Source: CAD feature listing. Evaluate the final solid. Frame: model axes, mm. A direction names the side the tool comes from. Give positions to 0.01 mm unless a question says otherwise; leave off trailing zeros. Write each loop counter-clockwise with the first axis right and the second up, starting at its lowest first coordinate (ties: lowest second). Pieces come first, ordered by that corner, then holes. Notation, with made-up numbers: (33.5, -14.5) -> (64.5, -14.5) arc R6 cw to (64.5, -10.5) -> close; hole circle Ø2 at (67, 28.25). An arc over 180 degrees is marked (long way). Write item = value, one per line.
from build123d import *

# Parameters (mm, degrees)
SKETCH_2_R               = 1.5
CUT_EXTRUDE_1_DEPTH      = 10
PATTERN_CIRCULAR_1_COUNT = 4
CUT_EXTRUDE_3_REACH      = 41.211
SKETCH_3_R               = 3.5
CUT_EXTRUDE_4_REACH      = 41.211
CUT_EXTRUDE_4_END_RADIUS = 1.5
SKETCH_4_W               = 31.367872694
SKETCH_4_H               = 2
CUT_EXTRUDE_START        = -24
SKETCH_5_W               = 2
SKETCH_5_H               = 28.424190946
CUT_EXTRUDE_5_DEPTH      = 24


with BuildPart() as part:
    # 草图1 → 旋转1 (revolve)
    with BuildSketch(Plane(origin=(0, 0, 0), x_dir=(0, 0, -1), z_dir=(1, 0, 0)), mode=Mode.PRIVATE) as revolve_1_sk:
        Polygon((-2.5, 6.5), (2.5, 6.5), (2.5, 9), (8.5, 9), (8.5, 0), (-26.5, 0), (-26.5, 9), (-22.5, 9), (-22.5, 12.5), (-2.5, 9.653578486), align=None)
    revolve(revolve_1_sk.sketch.rotate(Axis((0, 0, 115.12599891), (0, 0, -1)), 90), axis=Axis((0, 0, 115.12599891), (0, 0, -1)))

    # 草图2 → 切除-拉伸1 (cut)
    with BuildSketch(Plane(origin=(0, 0, 0), x_dir=(1, 0, 0), z_dir=(0, 1, 0))):
        with Locations(Location((0, 0, 0), (0, 0, 270))):
            Circle(SKETCH_2_R)
    cut_extrude_1 = extrude(amount=-CUT_EXTRUDE_1_DEPTH, mode=Mode.SUBTRACT)

    # 阵列(圆周)1: 切除-拉伸1 ×4 about axis
    pattern_circular_1_axis = Axis((0, 0, 2.5), (0, 0, 1))
    for i in range(1, PATTERN_CIRCULAR_1_COUNT):
        add(cut_extrude_1.rotate(pattern_circular_1_axis, i * 360 / PATTERN_CIRCULAR_1_COUNT), mode=Mode.SUBTRACT)

    # 草图3 → 切除-拉伸3 (cut, up to next)
    with BuildSketch(Plane(origin=(0, 0, -8.5), x_dir=(-1, 0, 0), z_dir=(0, 0, -1)), mode=Mode.PRIVATE) as cut_extrude_3_sk1:
        Circle(SKETCH_3_R)
    cut_extrude_3_tool1 = extrude(cut_extrude_3_sk1.sketch, amount=-CUT_EXTRUDE_3_REACH, mode=Mode.PRIVATE) & part.part
    add(cut_extrude_3_tool1.solids().sort_by_distance((0, 0, -8.5))[0], mode=Mode.SUBTRACT)

    # 切除-拉伸4: up to this cylinder (the profile starts outside it)
    cut_extrude_4_end = Plane(origin=(0, 0, 0), z_dir=(-1, 0, 0)) * Cylinder(CUT_EXTRUDE_4_END_RADIUS, 86.422, mode=Mode.PRIVATE)
    # 草图4 → 切除-拉伸4 (cut, up to the surface)
    with BuildSketch(Plane.XY.offset(26.5), mode=Mode.PRIVATE) as cut_extrude_4_sk1:
        Rectangle(SKETCH_4_W, SKETCH_4_H)
    cut_extrude_4_tool1 = extrude(cut_extrude_4_sk1.sketch, amount=-CUT_EXTRUDE_4_REACH, mode=Mode.PRIVATE) - cut_extrude_4_end
    add(cut_extrude_4_tool1.solids().sort_by_distance((0, 0, 26.5))[0], mode=Mode.SUBTRACT)

    # 草图5 → 切除-拉伸5 (cut)
    with BuildSketch(Plane.XY.offset(26.5).offset(CUT_EXTRUDE_START)):
        Rectangle(SKETCH_5_W, SKETCH_5_H)
    extrude(amount=CUT_EXTRUDE_5_DEPTH, mode=Mode.SUBTRACT)


solid = part.part
(1) Section query A-A (x = 0). Return loops of the section in (y, z).
Values follow:
outline = (-9, -8.5) -> (-3.5, -8.5) -> (-3.5, -1.5) -> (-6.5, -1.5) -> (-6.5, -2.5) -> (-9, -2.5) -> close; (-6.5, 1.5) -> (-3.5, 1.5) -> (-3.5, 2.5) -> (-6.5, 2.5) -> close; (3.5, -8.5) -> (9, -8.5) -> (9, -2.5) -> (6.5, -2.5) -> (6.5, -1.5) -> (3.5, -1.5) -> close; (3.5, 1.5) -> (6.5, 1.5) -> (6.5, 2.5) -> (3.5, 2.5) -> close
(2) First-contact query: pin 1 (4 mm diameter, centred on x = 0, z = 0, fed in from +Y); pin 2 (1.5 mm diameter, centred on x = 2.5, z = 12.5, fed in from -Y); pin 3 (3.5 mm diameter, centred on y = 0, z = 0, fed in from -X). Flat tips, straight axial feed; report the tip coordinate or a pass-through.
Values follow:
pin_1 = 6.5
pin_2 = -10.98
pin_3 = -6.5
(3) Section query D-D (y = -7.25). Give the number of separate pieces and of enclosed holes in the cut face, plus the area to 3 significant figures.
Values follow:
separate_pieces = 3
enclosed_holes = 0
area = 392 mm2
(4) Section query C-C (z = 0). Return loops of the section in (x, y), plus the area to 3 significant figures.
Values follow:
outline = (-6.32, -1.5) arc R6.5 ccw to (-1.5, -6.32) -> (-1.5, -3.16) arc R3.5 cw to (-3.16, -1.5) -> close; (-6.32, 1.5) -> (-3.16, 1.5) arc R3.5 cw to (-1.5, 3.16) -> (-1.5, 6.32) arc R6.5 ccw to start; (1.5, -6.32) arc R6.5 ccw to (6.32, -1.5) -> (3.16, -1.5) arc R3.5 cw to (1.5, -3.16) -> close; (1.5, 3.16) arc R3.5 cw to (3.16, 1.5) -> (6.32, 1.5) arc R6.5 ccw to (1.5, 6.32) -> close
area = 57.6 mm2
(5) Access query for faces 1 (the face through (0, -5, 2.5)), 2 (the face through (-3, 6, -2.5)), 3 (the face through (7, 1, 14)), 4 (the face through (5, -5, 2.5)), 5 (the face through (-6.633, -6.083, -5.542)). Directions: +Z, -Z, +X, -X, +Y, -Y. A direction counts if a zero-diameter tool reaches every point of the face in a straight line with its end or side. Return the directions, or none.
Values follow:
face_1 = +Z, +Y, -Y
face_2 = none
face_3 = +Z, +X, -X
face_4 = +X, -Y
face_5 = -Z
(6) Pull-direction query (Z, two-part tool) for faces 6 (the face through (1.265, 4.857, 0.806)), 7 (the face through (-7, -7, 22.5)), 8 (the face through (-1, -7, 14)); classes: pulls with the +Z half, pulls with the -Z half, needs draft (parallel to the pull), parting line crosses it, or undercut.
Values follow:
face_6 = undercut
face_7 = pulls with the +Z half
face_8 = needs draft
(7) Material intervals for line 1 (Z direction, x = -2.25, y = 8); line 2 (Z direction, x = 2.5, y = 9); line 3 (X direction, y = -3.5, z = 14), sorted ascending.
Values follow:
line_1 = -8.5 to -2.5, 2.5 to 26.5
line_2 = 2.5 to 22.5
line_3 = -10.73 to -1, 1 to 10.73
(8) Section query B-B (y = 0). Return loops of the section in (x, z).
Values follow:
outline = (-9, -8.5) -> (-3.5, -8.5) -> (-3.5, -1.5) -> (-6.5, -1.5) -> (-6.5, -2.5) -> (-9, -2.5) -> close; (3.5, -8.5) -> (9, -8.5) -> (9, -2.5) -> (6.5, -2.5) -> (6.5, -1.5) -> (3.5, -1.5) -> close
